from build123d import *

# Parameters (mm, degrees)
SKETCH1_W           = 50
SKETCH1_H           = 20
SKETCH1_R           = 1.75
BOSS_EXTRUDE1_DEPTH = 1.6
SKETCH3_R           = 0.375
CUT_EXTRUDE1_DEPTH  = 2.6
SKETCH2_W           = 0.3
SKETCH2_H           = 20
SKETCH2_W_2         = 1.5
SKETCH2_H_2         = 0.3
CUT_EXTRUDE2_DEPTH  = 0.6


with BuildPart() as part:
    # Sketch1 → Boss-Extrude1 (new body)
    with BuildSketch(Plane(origin=(0, 0, 0), x_dir=(1, 0, 0), z_dir=(0, 1, 0))):
        with Locations((25, 10)):
            Rectangle(SKETCH1_W, SKETCH1_H)
        with Locations((3, 17)):
            Circle(SKETCH1_R, mode=Mode.SUBTRACT)
        with Locations((47, 3)):
            Circle(SKETCH1_R, mode=Mode.SUBTRACT)
        with Locations((3, 3)):
            Circle(SKETCH1_R, mode=Mode.SUBTRACT)
        with Locations((47, 17)):
            Circle(SKETCH1_R, mode=Mode.SUBTRACT)
    extrude(amount=BOSS_EXTRUDE1_DEPTH)

    # Sketch3 → Cut-Extrude1 (cut, through all)
    with BuildSketch(Plane(origin=(0, 1.6, 0), x_dir=(1, 0, 0), z_dir=(0, 1, 0))):
        with Locations((8.25, 0.75)):
            Circle(SKETCH3_R)
        with Locations((9.75, 0.75)):
            Circle(SKETCH3_R)
        with Locations((9.75, 5.5)):
            Circle(SKETCH3_R)
        with Locations((9.75, 14.5)):
            Circle(SKETCH3_R)
    extrude(amount=-CUT_EXTRUDE1_DEPTH, mode=Mode.SUBTRACT)

    # Sketch2 → Cut-Extrude2 (cut)
    with BuildSketch(Plane(origin=(0, 1.6, 0), x_dir=(1, 0, 0), z_dir=(0, 1, 0))):
        Polygon((9.15, 0), (9.15, 19.65), (7.5, 19.65), (7.5, 19.35), (8.85, 19.35), (8.85, 0), align=None)
        with Locations((7.5, 10)):
            Rectangle(SKETCH2_W, SKETCH2_H)
        with Locations((10.5, 10)):
            Rectangle(SKETCH2_W, SKETCH2_H)
        with Locations((9.75, 10)):
            Rectangle(SKETCH2_W_2, SKETCH2_H_2)
    extrude(amount=-CUT_EXTRUDE2_DEPTH, mode=Mode.SUBTRACT)


solid = part.part
Input: part model. Units: mm. Frame: model coordinates. Coordinates: 2 decimals unless noted, no trailing zeros. Order: outer loops, then holes, each group sorted by start corner. A loop starts at its lowest first (then second) coordinate and runs counter-clockwise, first axis right, second up.
1. Contact query for a flat-ended pin moving along its axis: P1, Ø2, axis at x = 3, z = -17, coming from the -Y side. Output: stop coordinate, or through.
Checked values:
P1: passes through
2. Draft query along X for faces 1 (the flat face through (30, 1.6, -10)), 2 (the flat face through (0, 1, -10)), 3 (the cylindrical face through (48.669, 0.789, -17.526)). Return one class per face: +X half, -X half, draft (parallel to the pull), parting line (faces both ways), or undercut.
Checked values:
face 1: draft
face 2: -X half
face 3: undercut
3. Cut plane C-C, the plane y = 0.65. Count the separate pieces of the cut face and the enclosed holes in it, plus the area to 3 significant figures.
Checked values:
separate pieces: 1
enclosed holes: 8
area: 960 mm2
4. Ray query, line 1 along Z through (x, y) = (9.75, 0.95) (3 decimals); line 2 along X through (y, z) = (0.3, -17); line 3 along X through (y, z) = (1.15, -13). Return the intervals inside material, ascending.
Checked values:
line 1: z = -20 to -14.875, -14.125 to -5.875, -5.125 to -1.125, -0.375 to 0
line 2: x = 0 to 1.25, 4.75 to 45.25, 48.75 to 50
line 3: x = 0 to 7.35, 7.65 to 8.85, 9.15 to 10.35, 10.65 to 50
5. Cut plane B-B, the plane z = -17. Return loops of the section in (x, y).
Checked values:
outline: (0, 0) - (1.25, 0) - (1.25, 1.6) - (0, 1.6) - close; (4.75, 0) - (45.25, 0) - (45.25, 1.6) - (10.65, 1.6) - (10.65, 1) - (10.35, 1) - (10.35, 1.6) - (9.15, 1.6) - (9.15, 1) - (8.85, 1) - (8.85, 1.6) - (7.65, 1.6) - (7.65, 1) - (7.35, 1) - (7.35, 1.6) - (4.75, 1.6) - close; (48.75, 0) - (50, 0) - (50, 1.6) - (48.75, 1.6) - close
6. Cut plane A-A, the plane x = 47. Return loops of the section in (y, z).
Checked values:
outline: (0, -20) - (1.6, -20) - (1.6, -18.75) - (0, -18.75) - close; (0, -15.25) - (1.6, -15.25) - (1.6, -4.75) - (0, -4.75) - close; (0, -1.25) - (1.6, -1.25) - (1.6, 0) - (0, 0) - close
